Source: three-view drawing plus pictorial views. Frame: mm from the lowest corner of the part. A direction names the side the tool comes from. Coordinates: 2 decimals unless noted, no trailing zeros. Write each loop counter-clockwise with the first axis right and the second up, starting at its lowest first coordinate (ties: lowest second). Pieces come first, ordered by that corner, then holes. Notation, with made-up numbers: (75, 77.5) - (102, 77.5) arc R25 ccw to (102, 93.5) - close; hole circle Ø4 at (16.25, 45). An arc over 180 degrees is marked (long way). Answer as a JSON object with one key per item and string values. Group by question number.
Item 1: Mould query, pull axis X, two halves, no side actions, for the marked faces 1, 2 and 3. Classes: pulls with the +X half, pulls with the -X half, needs draft (parallel to the pull), parting line crosses it, or undercut.
Item 2: Line query: line 1 along Y through (x, z) = (3, 9.25); line 2 along Y through (x, z) = (17.5, 3); line 3 along X through (y, z) = (21, 1). Output: solid intervals per line, ascending. Write a range as from..to.
Item 3: Section A-A on x = 37. Return loops of the section in (y, z).
Item 4: Set-up query: the marked faces 4, 5 and 6. Return all of +Z, -Z, +X, -X, +Y, -Y with unobstructed straight access to the full face (end or side cutting, diameter ignored); none if empty.
Item 5: First-contact query: pin 1 Ø5 at (y, z) = (33, 14) entering from -X; pin 2 Ø5.5 at (x, z) = (50.57, 13.88) entering from -Y; pin 3 Ø6 at (x, z) = (9.5, 4.5) entering from +Y; pin 4 Ø1.5 at (x, y) = (47.5, 20) entering from +Z. Flat tips, straight axial feed; report the tip coordinate or a pass-through.
Item 6: Section D-D on x = 17.5. Return loops of the section in (y, z).
Item 7: Section B-B on z = 9.25. Return loops of the section in (x, y).
Item 8: Section C-C on y = 16. Return loops of the section in (x, z), and give its area (3 significant figures).
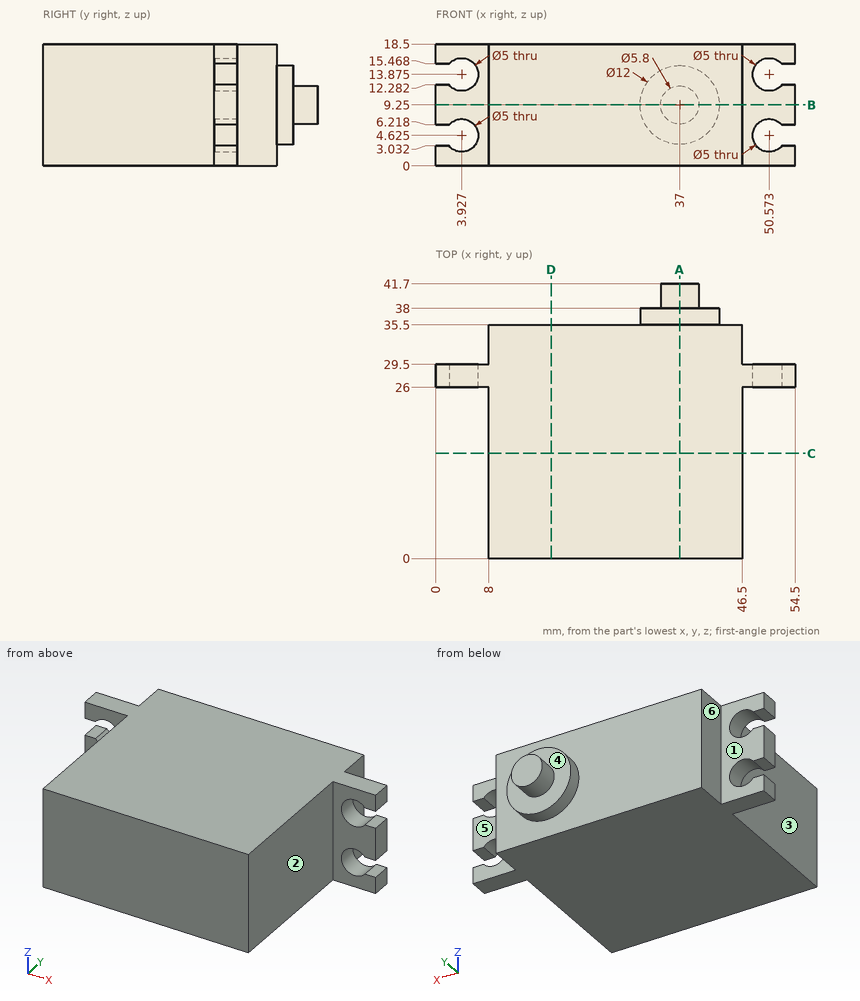
Checks:
{
 "1": {"face 1": "needs draft", "face 2": "pulls with the +X half", "face 3": "pulls with the -X half"},
 "2": {"line 1": "26..29.5", "line 2": "0..35.5", "line 3": "8..46.5"},
 "3": {"outline": "(0, 0) - (35.5, 0) - (35.5, 3.25) - (38, 3.25) - (38, 6.35) - (41.7, 6.35) - (41.7, 12.15) - (38, 12.15) - (38, 15.25) - (35.5, 15.25) - (35.5, 18.5) - (0, 18.5) - close"},
 "4": {"face 4": "+Y", "face 5": "+Z, -Z, +X, +Y", "face 6": "+Z, -Z, -X, +Y"},
 "5": {"pin 1": "x = 8", "pin 2": "y = 26", "pin 3": "y = 35.5", "pin 4": "through"},
 "6": {"outline": "(0, 0) - (35.5, 0) - (35.5, 18.5) - (0, 18.5) - close"},
 "7": {"outline": "(0, 26) - (8, 26) - (8, 0) - (46.5, 0) - (46.5, 26) - (54.5, 26) - (54.5, 29.5) - (46.5, 29.5) - (46.5, 35.5) - (43, 35.5) - (43, 38) - (39.9, 38) - (39.9, 41.7) - (34.1, 41.7) - (34.1, 38) - (31, 38) - (31, 35.5) - (8, 35.5) - (8, 29.5) - (0, 29.5) - close"},
 "8": {"outline": "(8, 0) - (46.5, 0) - (46.5, 18.5) - (8, 18.5) - close", "area": "712 mm^2"}
}
